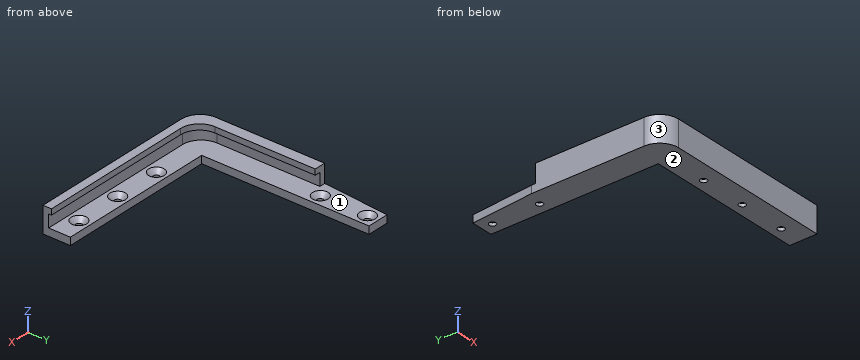
Autodesk Inventor part; units mm, degrees
ref_plane "YZ Plane" through (0, 0, 0) normal (1, 0, 0) x (0, 1, 0)
ref_plane "XZ Plane" through (0, 0, 0) normal (0, 1, 0) x (-1, 0, 0)
ref_plane "XY Plane" through (0, 0, 0) normal (0, 0, 1) x (1, 0, 0)
sketch "Sketch1" plane through (0, 0, 0) normal (0, 0, 1) x (1, 0, 0)
  circle A0 centre (120.7, -158.2779) radius 1.75
  circle A1 centre (95.7, -158.2779) radius 1.75
  circle A2 centre (70.7, -158.2779) radius 1.75
  circle A3 centre (17.5, -69.45) radius 1.75
  circle A4 centre (17.5, -94.45) radius 1.75
  line L0 (135.7, -152.5058) -> (135.7, -164.0501) construction
  circle A5 centre (45.7, -158.2779) radius 1.75
  line L1 (0, 0) -> (135.7, 0) construction
  line L2 (135.7, 0) -> (135.7, -9.1902) construction
  circle A6 centre (125.7, -4.5951) radius 1.75 construction
  circle A7 centre (115.7, -4.5951) radius 1.75 construction
  line L3 (-18.071, -149.5998) -> (178.1747, -149.5998) construction
  line L4 (23.9, 14.4501) -> (135.7, 14.4501)
  line L5 (135.7, 14.4501) -> (135.7, -164.0499)
  line L6 (135.7, -164.0499) -> (23.9, -164.0499)
  line L7 (11.9, -152.0499) -> (11.9, 2.4501)
  arc A8 (23.9, 14.4501) -> (11.9, 2.4501) centre (23.9, 2.4501) ccw
  arc A9 (11.9, -152.0499) -> (23.9, -164.0499) centre (23.9, -152.0499) ccw construction
  line L8 (11.9, -20.5499) -> (8.9, -20.5499)
  line L9 (8.9, -20.5499) -> (8.9, -164.0499)
  line L10 (8.9, -164.0499) -> (11.9, -164.0499)
  line L11 (11.9, -154.0499) -> (11.9, -20.5499)
  line L12 (8.9, -55.2999) -> (11.9, -55.2999)
  line L13 (11.9, -55.2999) -> (11.9, -94.2999)
  line L14 (11.9, -94.2999) -> (8.9, -94.2999)
  line L15 (8.9, -94.2999) -> (8.9, -55.2999)
  line L16 (21.9, -164.0499) -> (135.7, -164.0499)
  line L17 (135.7, -164.0499) -> (135.7, -167.0499)
  line L18 (135.7, -167.0499) -> (8.9, -167.0499)
  line L19 (8.9, -167.0499) -> (8.9, -164.0499)
  arc A10 (11.9, -154.0499) -> (21.9, -164.0499) centre (21.9, -154.0499) ccw
  line L20 (8.9, -20.5499) -> (23.5, -20.5499)
  line L21 (23.5, -167.0499) -> (8.9, -167.0499)
  line L22 (8.9, -167.0499) -> (8.9, -20.5499)
  line L23 (135.7, -138.0558) -> (135.7, -164.0499)
  line L24 (135.7, -164.0499) -> (11.9, -164.0499)
  line L25 (11.9, -164.0499) -> (11.9, -138.0558)
  line L26 (23.5, -20.5499) -> (23.5, -138.0558)
  line L27 (23.5, -149.5998) -> (23.5, -167.0499)
  line L28 (130.7, -138.0558) -> (130.7, -167.0499)
  line L29 (130.7, -167.0499) -> (135.7, -167.0499)
  line L30 (135.7, -167.0499) -> (135.7, -138.0558)
  line L31 (-26.1104, -138.0558) -> (23.5, -138.0558) construction
  line L32 (135.7, -138.0558) -> (178.6938, -138.0558) construction
  circle A11 centre (118.0205, -143.8278) radius 1.75 construction
  line L33 (130.7, -138.0558) -> (130.7, -152.5059)
  line L34 (130.7, -152.5059) -> (23.5, -152.5059)
  line L35 (23.5, -152.5059) -> (23.5, -138.0558)
  point P0 (20.72, -105.8556)
  point P1 (11.9, -164.0499)
  dimension "d0" = 3.5
  dimension "d1" = 3.5
  dimension "d2" = 3.5
  dimension "d3" = 3.5
  dimension "d4" = 3.5
  dimension "d5" = 15
  dimension "d6" = 25
  dimension "d7" = 25
  dimension "d8" = 3.5
  dimension "d9" = 25
  dimension "d10" = 69.45
  dimension "d11" = 25
  dimension "d13" = 3.5
  dimension "d14" = 3.5
  dimension "d15" = 10
  dimension "d16" = 10
  dimension "d17" = 17.5
  dimension "d18" = 0
  dimension "d20" = 123.8
  dimension "d21" = 178.5
  dimension "d22" = 149.5999
  dimension "d23" = 12
  dimension "d26" = 14.4501
  dimension "d27" = 0
  dimension "d28" = 0
  dimension "d29" = 135.7
  dimension "d30" = 3
  dimension "d31" = 35
  dimension "d32" = 0
  dimension "d33" = 3
  dimension "d34" = 39
  dimension "d35" = 69.75
  dimension "d36" = 3
  dimension "d37" = 0
  dimension "d38" = 10
  dimension "d46" = 5
  dimension "d72" = 5.772
  dimension "d73" = 3.5
  dimension "d74" = 5.772
  dimension "d75" = 14.4501
  dimension "d76" = 5.772
extrude "Extrusion1" add sketch "Sketch1" along normal blind 4 contours A0 | L20 L26 L35 L27 L16 A10 L11 L7 | L7 L12 L9 L8 | L28 L18 L27 L16 L6 | L6 L16 L27 L34 L28 | L7 L11 L25 L10 L9 L14 | L27 L18 L19 L10 L24 L16 | L24 L25 A10
chamfer "Chamfer1" distance 2.4 angle 45 5 edges at (15.75, -69.45, 4) (15.75, -94.45, 4) (43.95, -158.2779, 4) (68.95, -158.2779, 4) (93.95, -158.2779, 4)
sketch "Sketch2" plane through (0, 0, 4) normal (0, 0, 1) x (1, 0, 0)
  line L0 (8.9, -20.5499) -> (8.9, -55.2999)
  line L1 (11.9, -94.2999) -> (11.9, -55.2999)
  line L2 (8.9, -20.5499) -> (11.9, -20.5499)
  line L3 (11.9, -20.5499) -> (11.9, -55.2999)
  line L4 (11.9, -55.2999) -> (8.9, -55.2999)
  line L5 (8.9, -55.2999) -> (8.9, -20.5499)
  line L6 (8.9, -94.2999) -> (8.9, -167.0499)
  line L7 (8.9, -167.0499) -> (130.7, -167.0499)
  line L8 (8.9, -94.2999) -> (11.9, -94.2999)
  line L9 (11.9, -94.2999) -> (11.9, -167.0499)
  line L10 (11.9, -167.0499) -> (8.9, -167.0499)
  line L11 (8.9, -167.0499) -> (8.9, -94.2999)
  line L12 (130.7, -167.0499) -> (11.9, -167.0499)
  line L13 (11.9, -167.0499) -> (11.9, -164.0499)
  line L14 (11.9, -164.0499) -> (130.7, -164.0499)
  line L15 (130.7, -164.0499) -> (130.7, -167.0499)
  point P0 (0, 0)
  dimension "d47" = 3
extrude "Extrusion2" add sketch "Sketch2" along normal blind 9.7
sketch "Sketch3" plane through (0, 0, 13.7) normal (0, 0, 1) x (1, 0, 0)
  line L0 (8.9, -94.2999) -> (8.9, -167.0499)
  line L1 (8.9, -167.0499) -> (130.7, -167.0499)
  line L2 (8.9, -94.2999) -> (14.9, -94.2999)
  line L3 (14.9, -94.2999) -> (14.9, -152.5499)
  line L4 (14.9, -167.0499) -> (8.9, -167.0499)
  line L5 (8.9, -167.0499) -> (8.9, -94.2999)
  line L6 (130.7, -167.0499) -> (14.9, -167.0499)
  line L7 (14.9, -167.0499) -> (14.9, -162.5499)
  line L8 (24.9, -162.5499) -> (130.7, -162.5499)
  line L9 (130.7, -162.5499) -> (130.7, -167.0499)
  line L10 (8.9, -20.5499) -> (8.9, -55.2999)
  line L11 (8.9, -20.5499) -> (14.9, -20.5499)
  line L12 (14.9, -20.5499) -> (14.9, -55.2999)
  line L13 (14.9, -55.2999) -> (8.9, -55.2999)
  line L14 (8.9, -55.2999) -> (8.9, -20.5499)
  arc A0 (14.9, -152.5499) -> (24.9, -162.5499) centre (24.9, -152.5499) ccw
  point P0 (0, 0)
  dimension "d50" = 6
  dimension "d51" = 4.5
  dimension "d52" = 6
  dimension "d53" = 10
extrude "Extrusion3" add sketch "Sketch3" against normal blind 3
sketch "Sketch4" plane through (0, 0, 13.7) normal (0, 0, 1) x (1, 0, 0)
  line L0 (130.7, -164.0499) -> (130.7, -152.5059)
  line L1 (130.7, -138.0558) -> (108.2, -138.0558)
  line L2 (108.2, -138.0558) -> (108.2, -174.4864)
  line L3 (108.2, -174.4864) -> (130.7, -174.4864)
  line L4 (130.7, -174.4864) -> (130.7, -138.0558)
  line L5 (-4.6471, -18.4715) -> (48.1424, -18.4715)
  line L6 (48.1424, -18.4715) -> (48.1424, -63.678)
  line L7 (48.1424, -63.678) -> (-4.6471, -63.678)
  line L8 (-4.6471, -63.678) -> (-4.6471, -18.4715)
  circle A0 centre (17.5, -69.45) radius 4.15
  circle A1 centre (17.5, -69.45) radius 0.7081
  point P0 (0, 0)
  dimension "d62" = 22.5
  dimension "d79" = 5.772
extrude "Extrusion5" cut sketch "Sketch4" against normal blind 22.05 contours L4 L3 L2 L1 L0 | L5 L6 L7 L8
sketch "Sketch5" plane through (0, 0, 13.7) normal (0, 0, 1) x (1, 0, 0)
  line L0 (-3.6304, -50.2999) -> (31.4299, -50.2999)
  line L1 (31.4299, -50.2999) -> (31.4299, -99.2999)
  line L2 (31.4299, -99.2999) -> (-3.6304, -99.2999)
  line L3 (-3.6304, -99.2999) -> (-3.6304, -50.2999)
  line L4 (8.9, -55.2999) -> (14.9, -55.2999)
  line L5 (14.9, -94.2999) -> (8.9, -94.2999)
  point P0 (0, 0)
  dimension "d67" = 5
  dimension "d68" = 5
extrude "Extrusion6" cut sketch "Sketch5" against normal up to surface (9.7 mm away)
fillet "Fillet1" radius 10 1 edges at (8.9, -167.0499, 6.85)
fillet "Fillet2" radius 10 1 edges at (11.9, -164.0499, 7.35)
chamfer "Chamfer3" distance 3 angle 45 1 edges at (8.9, -94.2999, 2)
sketch "Sketch6" plane through (0, 0, 4) normal (0, 0, 1) x (1, 0, 0)
  line L0 (11.9, -63.678) -> (11.9, -94.2999)
  line L1 (8.9, -97.2999) -> (11.9, -94.2999)
  line L2 (11.9, -63.678) -> (8.9, -97.2999)
  line L3 (8.9, -97.2999) -> (11.9, -94.2999)
  line L4 (11.9, -94.2999) -> (11.9, -63.678)
  point P0 (0, 0)
extrude "Extrusion7" add sketch "Sketch6" against normal up to surface (4 mm away)
equation "\"d26\" = -0.5 * d22 + 0.5 * d21"
equation "\"d35\" = -0.5 * d34 + 0.5 * d21"
equation "\"d39\" = d19"
properties part number "iPadGolf6HolderMount"
CAD build for the part. Positions are in the model's coordinates, mm. Face numbers are marked on the shaded views. Round coordinates to 2 decimals unless told otherwise and drop trailing zeros. Order: outer loops, then holes, each group sorted by start corner. A loop starts at its lowest first (then second) coordinate and runs counter-clockwise, first axis right, second up. Notation, with made-up numbers: (-6, 24.25) -> (29, 24.25) arc R29 ccw to (29, 49.25) -> close; hole circle Ø10 at (5.25, 33.5). An arc over 180 degrees is marked (long way). Write item = value, one per line.
(1) Cut at C-C (y = -136.5). Write the cut outline in (x, z).
Answers follow:
outline = (8.9, 0) -> (23.5, 0) -> (23.5, 4) -> (11.9, 4) -> (11.9, 10.7) -> (14.9, 10.7) -> (14.9, 13.7) -> (8.9, 13.7) -> close
(2) Flat gauge pins, fed straight in: P1, Ø3.5, axis at x = 73.5, z = 11.5, coming from the +Y side; P2, Ø4.5, axis at x = 70.7, y = -158.28, coming from the -Z side; P3, Ø8, axis at y = -116, z = 10.5, coming from the +X side; P4, Ø3, axis at x = 12.5, z = 10.5, coming from the +Y side. Where does each tip first touch, or does it go through?
Answers follow:
P1 = -162.55
P2 = 0
P3 = 14.9
P4 = -99.3
(3) Cut at A-A (x = 45.7). Write the cut outline in (y, z), plus the area to 3 significant figures.
Answers follow:
outline = (-167.05, 0) -> (-160.03, 0) -> (-160.03, 1.6) -> (-162.43, 4) -> (-164.05, 4) -> (-164.05, 10.7) -> (-162.55, 10.7) -> (-162.55, 13.7) -> (-167.05, 13.7) -> close; (-156.53, 0) -> (-152.51, 0) -> (-152.51, 4) -> (-154.13, 4) -> (-156.53, 1.6) -> close
area = 72.0 mm²
(4) Cut at B-B (y = -94.45). Write the cut outline in (x, z).
Answers follow:
outline = (9.15, 0) -> (15.75, 0) -> (15.75, 1.6) -> (13.35, 4) -> (9.15, 4) -> close; (19.25, 0) -> (23.5, 0) -> (23.5, 4) -> (21.65, 4) -> (19.25, 1.6) -> close
(5) Pull direction Z, two halves, no side cores. Call the marked faces 1, 2 and 3: +Z half, -Z half, draft (parallel to the pull), parting line (faces both ways), or undercut.
Answers follow:
face_1 = undercut
face_2 = -Z half
face_3 = draft
(6) Cut at D-D (z = 12). Write the cut outline in (x, y).
Answers follow:
outline = (8.9, -157.05) arc R10 ccw to (18.9, -167.05) -> (108.2, -167.05) -> (108.2, -162.55) -> (24.9, -162.55) arc R10 cw to (14.9, -152.55) -> (14.9, -99.3) -> (8.9, -99.3) -> close
(7) Drill centre lines: L1, parallel to Y at x = 95.7, z = 0.55; L2, parallel to Y at x = 17.5, z = 0.6; L3, parallel to Y at x = 76, z = 1.5. Where is each one in solid material? Low to high.
Answers follow:
L1 = -167.05 to -160.03, -156.53 to -152.51
L2 = -166.95 to -96.2, -92.7 to -71.2, -67.7 to -63.68
L3 = -167.05 to -152.51
